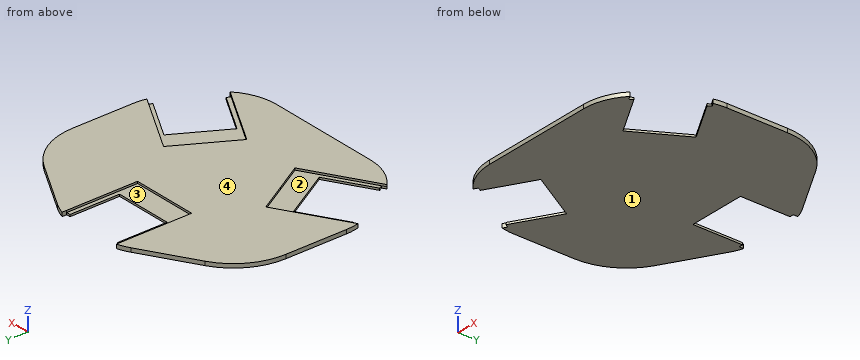
Solid Edge part; units mm, degrees
sketch "Sketch1" plane through (0, 0, 0) normal (0, 0, 1) x (1, 0, 0)
  line L0 (56.0106, 155.6218) -> (122.779, 117.073)
  arc A0 (122.779, 117.073) -> (162.779, 47.791) centre (82.779, 47.791) cw
  line L1 (162.779, -29.3066) -> (162.779, 47.791)
  arc A1 (153.4008, -64.3066) -> (162.779, -29.3066) centre (92.779, -29.3066) ccw
  line L2 (142.8955, -82.5023) -> (153.4008, -64.3066)
  line L3 (142.8955, -82.5023) -> (132.3902, -100.698)
  arc A2 (132.3902, -100.698) -> (106.7685, -126.3198) centre (71.7685, -65.698) cw
  arc A3 (106.7685, -126.3198) -> (71.7685, -135.698) centre (71.7685, -65.698) cw
  line L4 (-71.7658, -135.698) -> (71.7685, -135.698)
  arc A4 (-106.7658, -126.3198) -> (-71.7658, -135.698) centre (-71.7658, -65.698) ccw
  arc A5 (-132.3876, -100.698) -> (-106.7658, -126.3198) centre (-71.7658, -65.698) ccw
  line L5 (-153.3995, -64.3043) -> (-132.3876, -100.698)
  arc A6 (-153.3995, -64.3043) -> (-162.7777, -29.3043) centre (-92.7777, -29.3043) cw
  line L6 (-162.7777, -29.3043) -> (-162.7777, 47.7933)
  arc A7 (-122.779, 117.073) -> (-162.7777, 47.7933) centre (-82.7804, 47.7933) ccw
  line L7 (-56.0106, 155.6218) -> (-122.779, 117.073)
  arc A8 (-21.0106, 165) -> (-56.0106, 155.6218) centre (-21.0106, 95) ccw
  line L8 (0, 165) -> (-21.0106, 165)
  line L9 (0, 165) -> (21.0106, 165)
  arc A9 (21.0106, 165) -> (56.0106, 155.6218) centre (21.0106, 95) cw
extrude "Protrusion1" add sketch "Sketch1" along normal blind 5
sketch "Sketch2" plane through (0.0007, 14.651, 5) normal (0, 0, 1) x (1, 0, 0)
  line L0 (-57.3742, -47.7772) -> (-36.7492, -83.5007)
  line L1 (-140.6722, -143.5007) -> (-36.7492, -83.5007)
  line L2 (-181.9222, -72.0536) -> (-140.6722, -143.5007)
  line L3 (-77.9992, -12.0536) -> (-181.9222, -72.0536)
  line L4 (-57.3742, -47.7772) -> (-77.9992, -12.0536)
  line L5 (140.6709, -143.5007) -> (36.7478, -83.5007)
  line L6 (57.3728, -47.7772) -> (36.7478, -83.5007)
  line L7 (57.3728, -47.7772) -> (77.9978, -12.0536)
  line L8 (77.9978, -12.0536) -> (181.9209, -72.0536)
  line L9 (181.9209, -72.0536) -> (140.6709, -143.5007)
  line L10 (-0.001, 51.599) -> (41.249, 51.5984)
  line L11 (41.249, 51.5984) -> (41.2508, 171.5984)
  line L12 (41.2508, 171.5984) -> (-41.2492, 171.5996)
  line L13 (-41.2492, 171.5996) -> (-41.251, 51.5996)
  line L14 (-0.001, 51.599) -> (-41.251, 51.5996)
extrude "ExtrudedCutout_4" cut sketch "Sketch2" against normal blind 2.5
sketch "Sketch3" plane through (0.0007, 14.651, 5) normal (0, 0, 1) x (1, 0, 0)
  line L0 (-62.6319, -92.6706) -> (-98.8819, -29.8837)
  line L1 (-153.4415, -61.3837) -> (-98.8819, -29.8837)
  line L2 (-153.4415, -61.3837) -> (-155.9415, -57.0536)
  line L3 (-155.9415, -57.0536) -> (-181.9222, -72.0536)
  line L4 (-181.9222, -72.0536) -> (-140.6722, -143.5007)
  line L5 (-140.6722, -143.5007) -> (-114.6915, -128.5007)
  line L6 (-114.6915, -128.5007) -> (-117.1915, -124.1706)
  line L7 (-117.1915, -124.1706) -> (-62.6319, -92.6706)
extrude "ExtrudedCutout_5" cut sketch "Sketch3" against normal blind 5
sketch "Sketch4" plane through (0.0007, 14.651, 5) normal (0, 0, 1) x (1, 0, 0)
  line L0 (41.2504, 141.5984) -> (41.2508, 171.5984)
  line L1 (41.2508, 171.5984) -> (-41.2492, 171.5996)
  line L2 (-41.2492, 171.5996) -> (-41.2496, 141.5996)
  line L3 (-41.2496, 141.5996) -> (-36.2496, 141.5996)
  line L4 (-36.2496, 141.5996) -> (-36.2506, 78.5996)
  line L5 (-36.2506, 78.5996) -> (36.2494, 78.5985)
  line L6 (36.2504, 141.5985) -> (36.2494, 78.5985)
  line L7 (36.2504, 141.5985) -> (41.2504, 141.5984)
  line L8 (153.4401, -61.3837) -> (98.8805, -29.8837)
  line L9 (62.6305, -92.6706) -> (98.8805, -29.8837)
  line L10 (117.1901, -124.1706) -> (62.6305, -92.6706)
  line L11 (117.1901, -124.1706) -> (114.6901, -128.5007)
  line L12 (140.6709, -143.5007) -> (114.6901, -128.5007)
  line L13 (181.9209, -72.0536) -> (140.6709, -143.5007)
  line L14 (155.9401, -57.0536) -> (181.9209, -72.0536)
  line L15 (153.4401, -61.3837) -> (155.9401, -57.0536)
extrude "ExtrudedCutout_6" cut sketch "Sketch4" against normal blind 5
properties material "Polycarbonate"
CAD build for the part. Positions are in the model's coordinates, mm. Face numbers are marked on the shaded views. A direction names the side the tool comes from. Give positions to 0.01 mm unless a question says otherwise; leave off trailing zeros. Order: outer loops, then holes, each group sorted by start corner. A loop starts at its lowest first (then second) coordinate and runs counter-clockwise, first axis right, second up. Notation, with made-up numbers: (8.25, -10.5) - (51.25, -10.5) arc R13 ccw to (51.25, -3.5) - close; hole circle Ø1 at (76, -34.75). An arc over 180 degrees is marked (long way). Answer in a Markdown table with one row per item.
1. Probe probe 1 along X at (y, z) = (-26.5, 3.15); probe 2 along Z at (x, y) = (-73, -57); probe 3 along X at (y, z) = (67.5, 3.85). List the from-to ranges inside material, lowest first. Write a range as [from, to].
Data:
| item | result |
|---|---|
| probe 1 | x = [-162.78, -128.4], [-61.2, 61.2], [128.4, 162.78] |
| probe 2 | z = [0, 2.5] |
| probe 3 | x = [-160.31, -41.25], [41.25, 160.31] |
2. Tool access for the marked faces 3 and 4: list every direction of +Z, -Z, +X, -X, +Y, -Y with a clear straight run to the whole face (end or side of a thin tool).
Data:
| item | result |
|---|---|
| face 3 | +Z, +Y |
| face 4 | +Z, +X, -X, +Y, -Y |
3. Saw through at C-C, the plane y = 85.5. Give the cut face in (x, z).
Data:
| item | result |
|---|---|
| outline | (-153.33, 0) - (153.33, 0) - (153.33, 5) - (41.25, 5) - (41.25, 2.5) - (-41.25, 2.5) - (-41.25, 5) - (-153.33, 5) - close |
4. Saw through at D-D, the plane x = -23. Give the cut face in (y, z).
Data:
| item | result |
|---|---|
| outline | (-135.7, 0) - (93.25, 0) - (93.25, 2.5) - (66.25, 2.5) - (66.25, 5) - (-135.7, 5) - close |
5. Pull direction Y, two halves, no side cores. Call the marked faces 1 and 2: pulls with the +Y half, pulls with the -Y half, needs draft (parallel to the pull), parting line crosses it, or undercut.
Data:
| item | result |
|---|---|
| face 1 | needs draft |
| face 2 | undercut |
6. Flat gauge pins, fed straight in: pin 1 (12 mm diameter, centred on x = 97.5, y = -4.5, fed in from -Z); pin 2 (0.8 mm diameter, centred on x = -4, z = 4, fed in from +Y); pin 3 (2 mm diameter, centred on y = 159.5, z = 1, fed in from +X); pin 4 (3 mm diameter, centred on y = 107, z = 3.5, fed in from +X). Where does each tip first touch, or does it go through?
Data:
| item | result |
|---|---|
| pin 1 | stops at z = 0 |
| pin 2 | stops at y = 66.25 |
| pin 3 | stops at x = 50.47 |
| pin 4 | stops at x = 138.18 |
7. Saw through at B-B, the plane y = 142. Give the cut face in (x, z), plus the area to 3 significant figures.
Data:
| item | result |
|---|---|
| outline | (-79.6, 0) - (-36.25, 0) - (-36.25, 2.5) - (-41.25, 2.5) - (-41.25, 5) - (-79.6, 5) - close; (36.25, 0) - (79.6, 0) - (79.6, 5) - (41.25, 5) - (41.25, 2.5) - (36.25, 2.5) - close |
| area | 409 mm² |
